```python
from build123d import *

# Parameters (mm, degrees)
SKETCH_2_R      = 35
SKETCH_2_W      = 10.5
SKETCH_2_H      = 10.5
EXTRUDE_1_DEPTH = 20


with BuildPart() as part:
    # Эскиз2 → Бобышка-Вытянуть1 (new body)
    with BuildSketch(Plane.XY):
        Circle(SKETCH_2_R)
        with BuildLine():
            ThreePointArc((-30.540010176, 11.115654658), (-32.006251973, 5.643565774), (-32.5, 0))
            Line((-32.5, 0), (-10, 0))
            ThreePointArc((-10, 0), (-9.84807753, 1.736481777), (-9.396926208, 3.420201433))
            Line((-9.396926208, 3.420201433), (-30.540010176, 11.115654658))
        make_face(mode=Mode.SUBTRACT)
        with BuildLine():
            ThreePointArc((-11.115654658, -30.540010176), (-5.643565774, -32.006251973), (0, -32.5))
            Line((0, -32.5), (0, -10))
            ThreePointArc((0, -10), (-1.736481777, -9.84807753), (-3.420201433, -9.396926208))
            Line((-3.420201433, -9.396926208), (-11.115654658, -30.540010176))
        make_face(mode=Mode.SUBTRACT)
        with BuildLine():
            ThreePointArc((30.540010176, -11.115654658), (32.006251973, -5.643565774), (32.5, 0))
            Line((32.5, 0), (10, 0))
            ThreePointArc((10, 0), (9.84807753, -1.736481777), (9.396926208, -3.420201433))
            Line((9.396926208, -3.420201433), (30.540010176, -11.115654658))
        make_face(mode=Mode.SUBTRACT)
        with BuildLine():
            ThreePointArc((-13.735093507, 29.455003079), (-18.641234181, 26.622441439), (-22.980970389, 22.980970389))
            Line((-22.980970389, 22.980970389), (-7.071067812, 7.071067812))
            ThreePointArc((-7.071067812, 7.071067812), (-5.735764364, 8.191520443), (-4.226182617, 9.06307787))
            Line((-4.226182617, 9.06307787), (-13.735093507, 29.455003079))
        make_face(mode=Mode.SUBTRACT)
        Rectangle(SKETCH_2_W, SKETCH_2_H, mode=Mode.SUBTRACT)
        with BuildLine():
            Line((0, 10), (0, 32.5))
            ThreePointArc((0, 32.5), (5.643565774, 32.006251973), (11.115654658, 30.540010176))
            Line((11.115654658, 30.540010176), (3.420201433, 9.396926208))
            ThreePointArc((3.420201433, 9.396926208), (1.736481777, 9.84807753), (0, 10))
        make_face(mode=Mode.SUBTRACT)
        with BuildLine():
            Line((9.06307787, 4.226182617), (29.455003079, 13.735093507))
            ThreePointArc((29.455003079, 13.735093507), (26.622441439, 18.641234181), (22.980970389, 22.980970389))
            Line((22.980970389, 22.980970389), (7.071067812, 7.071067812))
            ThreePointArc((7.071067812, 7.071067812), (8.191520443, 5.735764364), (9.06307787, 4.226182617))
        make_face(mode=Mode.SUBTRACT)
        with BuildLine():
            Line((4.226182617, -9.06307787), (13.735093507, -29.455003079))
            ThreePointArc((13.735093507, -29.455003079), (18.641234181, -26.622441439), (22.980970389, -22.980970389))
            Line((22.980970389, -22.980970389), (7.071067812, -7.071067812))
            ThreePointArc((7.071067812, -7.071067812), (5.735764364, -8.191520443), (4.226182617, -9.06307787))
        make_face(mode=Mode.SUBTRACT)
        with BuildLine():
            Line((-9.06307787, -4.226182617), (-29.455003079, -13.735093507))
            ThreePointArc((-29.455003079, -13.735093507), (-26.622441439, -18.641234181), (-22.980970389, -22.980970389))
            Line((-22.980970389, -22.980970389), (-7.071067812, -7.071067812))
            ThreePointArc((-7.071067812, -7.071067812), (-8.191520443, -5.735764364), (-9.06307787, -4.226182617))
        make_face(mode=Mode.SUBTRACT)
    extrude(amount=EXTRUDE_1_DEPTH)


solid = part.part
```
The listing builds one solid part. Answer for the finished solid, in the listing's coordinates (mm). A direction names the side the tool comes from. Coordinates: 2 decimals unless noted, no trailing zeros. Loops run counter-clockwise (first coordinate to the right, second up) from the corner with the lowest first, then second, coordinate; pieces in that order, holes last. Notation, with made-up numbers: (-26.75, -5.75) - (17.25, -5.75) arc R34 cw to (17.25, 29.25) - close; hole circle Ø9 at (87, 46). An arc over 180 degrees is marked (long way). Use a Markdown table: item, result. Add a question column.
1) Find the intervals of material crossed by line 1 (X direction, y = 21.5, z = 12); line 2 (X direction, y = -24, z = 8); line 3 (X direction, y = 17, z = 4.5), in increasing order.
2) The part is cut by section A-A, the plane y = 12. Give the vertices of the cut face in (x, z).
3) The part is cut by section C-C, the plane x = -20. Give the vertices of the cut face in (y, z).
4) For faces 3 (the flat face through (19.82, -7.214, 9.86)), 4 (the flat face through (7, 0, 0)), determine the directions among +Z, -Z, +X, -X, +Y, -Y from which every point of the face is accessible in a straight line to the end or side of a thin tool.
5) Given pin 1 (2 mm diameter, centred on x = 3, z = 8, fed in from -Y); pin 2 (1.5 mm diameter, centred on x = 16.5, z = 15.5, fed in from -Y); pin 3 (1 mm diameter, centred on y = 11, z = 10, fed in from -X), each flat-ended and moving along its own axis, determine where each tip first touches the part or whether it passes through.
6) The part is cut by section D-D, the plane z = 11. State how many separate pieces and enclosed holes the cut face has, and give its area (3 significant figures).
7) The mould has two halves that part along Y. Classify faces 1 (the flat face through (7, 0, 20)), 2 (the flat face through (8.914, -19.116, 9.86)): released by +Y, released by -Y, zero draft, split by the parting line, or undercut.
8) The part is cut by section B-B, the plane x = 27.5. Give the vertices of the cut face in (y, z).
Here are the results:
| question | item | result |
|---|---|---|
| 1 | line 1 | x = -27.62 to -21.5, -10.03 to 0, 7.83 to 21.5, 24.37 to 27.62 |
| 1 | line 2 | x = -25.48 to -8.74, 0 to 11.19, 21.91 to 25.48 |
| 1 | line 3 | x = -30.59 to -17, -7.93 to 0, 6.19 to 17, 27.7 to 30.59 |
| 2 | outline | (-32.88, 0) - (-12, 0) - (-12, 20) - (-32.88, 20) - close; (-5.6, 0) - (0, 0) - (0, 20) - (-5.6, 20) - close; (4.37, 0) - (12, 0) - (12, 20) - (4.37, 20) - close; (25.73, 0) - (32.88, 0) - (32.88, 20) - (25.73, 20) - close |
| 3 | outline | (-28.72, 0) - (-20, 0) - (-20, 20) - (-28.72, 20) - close; (-9.33, 0) - (0, 0) - (0, 20) - (-9.33, 20) - close; (7.28, 0) - (20, 0) - (20, 20) - (7.28, 20) - close; (25.62, 0) - (28.72, 0) - (28.72, 20) - (25.62, 20) - close |
| 4 | face 3 | +Z, -Z |
| 4 | face 4 | -Z, +X, -X, +Y, -Y |
| 5 | pin 1 | stops at y = -34.94 |
| 5 | pin 2 | stops at y = -31.26 |
| 5 | pin 3 | stops at x = -33.39 |
| 6 | separate pieces | 1 |
| 6 | enclosed holes | 9 |
| 6 | area | 2,400 mm^2 |
| 7 | face 1 | zero draft |
| 7 | face 2 | undercut |
| 8 | outline | (-21.65, 0) - (-10.01, 0) - (-10.01, 20) - (-21.65, 20) - close; (0, 0) - (12.82, 0) - (12.82, 20) - (0, 20) - close; (17.32, 0) - (21.65, 0) - (21.65, 20) - (17.32, 20) - close |
